```python
from build123d import *

# Parameters (mm, degrees)
SKETCH1_R           = 95.25
BOSS_EXTRUDE1_DEPTH = 19.05
SKETCH2_R           = 56.515
CUT_EXTRUDE1_DEPTH  = 19.05
SKETCH3_R           = 46.355
CUT_EXTRUDE2_DEPTH  = 19.05
SKETCH5_R           = 3.175
CUT_EXTRUDE3_DEPTH  = 38.1
CIRPATTERN1_COUNT   = 3
SKETCH6_R           = 3.175
CUT_EXTRUDE4_DEPTH  = 19.05
CIRPATTERN2_COUNT   = 3


with BuildPart() as part:
    # Sketch1 → Boss-Extrude1 (new body, symmetric)
    with BuildSketch(Plane(origin=(0, 0, 0), x_dir=(1, 0, 0), z_dir=(0, 1, 0))):
        Circle(SKETCH1_R)
    extrude(amount=BOSS_EXTRUDE1_DEPTH, both=True)

    # Sketch2 → Cut-Extrude1 (cut)
    with BuildSketch(Plane(origin=(0, 19.05, 0), x_dir=(-1, 0, 0), z_dir=(0, 1, 0))):
        Circle(SKETCH2_R)
    extrude(amount=-CUT_EXTRUDE1_DEPTH, mode=Mode.SUBTRACT)

    # Sketch3 → Cut-Extrude2 (cut)
    with BuildSketch(Plane.XZ.offset(19.05)):
        Circle(SKETCH3_R)
    extrude(amount=-CUT_EXTRUDE2_DEPTH, mode=Mode.SUBTRACT)

    # Sketch5 → Cut-Extrude3 (cut)
    with BuildSketch(Plane(origin=(0, 19.05, 0), x_dir=(-1, 0, 0), z_dir=(0, 1, 0))):
        with Locations((-76.2, 0)):
            Circle(SKETCH5_R)
    cut_extrude3 = extrude(amount=-CUT_EXTRUDE3_DEPTH, mode=Mode.SUBTRACT)

    # CirPattern1: Cut-Extrude3 ×3 about axis
    cirpattern1_axis = Axis((0, 0, 0), (0, 1, 0))
    for i in range(1, CIRPATTERN1_COUNT):
        add(cut_extrude3.rotate(cirpattern1_axis, i * 360 / CIRPATTERN1_COUNT), mode=Mode.SUBTRACT)

    # Sketch6 → Cut-Extrude4 (cut)
    with BuildSketch(Plane.XZ.offset(19.05)):
        with Locations((44.7675, 77.539584528)):
            Circle(SKETCH6_R)
    cut_extrude4 = extrude(amount=-CUT_EXTRUDE4_DEPTH, mode=Mode.SUBTRACT)

    # CirPattern2: Cut-Extrude4 ×3 about axis
    cirpattern2_axis = Axis((0, 0, 0), (0, 1, 0))
    for i in range(1, CIRPATTERN2_COUNT):
        add(cut_extrude4.rotate(cirpattern2_axis, i * 360 / CIRPATTERN2_COUNT), mode=Mode.SUBTRACT)


solid = part.part
```
Work out the finished part from the listing and answer in its coordinate system (mm). A direction names the side the tool comes from. Coordinates: 2 decimals unless noted, no trailing zeros. Write each loop counter-clockwise with the first axis right and the second up, starting at its lowest first coordinate (ties: lowest second). Pieces come first, ordered by that corner, then holes. Notation, with made-up numbers: (72, 6.5) - (83, 6.5) arc R16 ccw to (83, 24.5) - close; hole circle Ø1 at (-25.5, 35). An arc over 180 degrees is marked (long way). Answer as a JSON object with one key per item and string values.
Q1. Find section A-A (x = 0). Write down the section's boundary in (y, z) (3 decimals).
Results list:
{"outline": "(-19.05, -95.25) - (19.05, -95.25) - (19.05, -56.515) - (0, -56.515) - (0, -46.355) - (-19.05, -46.355) - close; (-19.05, 46.355) - (0, 46.355) - (0, 56.515) - (19.05, 56.515) - (19.05, 95.25) - (-19.05, 95.25) - close"}
Q2. Find section D-D (x = 76.2). Write down the section's boundary in (y, z) (3 decimals).
Results list:
{"outline": "(-19.05, -57.15) - (19.05, -57.15) - (19.05, -3.175) - (-19.05, -3.175) - close; (-19.05, 3.175) - (19.05, 3.175) - (19.05, 57.15) - (-19.05, 57.15) - close"}
Q3. Given pin 1 Ø7.5 at (x, z) = (-38.1, 65.99) entering from -Y; pin 2 Ø3 at (y, z) = (10, -36) entering from +X; pin 3 Ø6 at (y, z) = (15, -60) entering from -X; pin 4 Ø5 at (x, z) = (-89.5, 0.5) entering from -Y, each flat-ended and moving along its own axis, determine where each tip first touches the part or whether it passes through.
Results list:
{"pin 1": "stops at y = -19.05", "pin 2": "stops at x = 88.78", "pin 3": "stops at x = -76.31", "pin 4": "stops at y = 0"}
Q4. Consider L1, parallel to Z at x = -38, y = -1; L2, parallel to Z at x = -38.1, y = -9.5; L3, parallel to Z at x = 0, y = -14 (3 decimals). Determine where each line is inside the solid, lowest interval first. Write a range as from..to.
Results list:
{"L1": "z = -87.34..-69.16, -62.82..-26.55, 26.55..62.82, 69.16..87.34", "L2": "z = -87.3..-69.17, -62.82..-26.4, 26.4..62.82, 69.17..87.3", "L3": "z = -95.25..-46.355, 46.355..95.25"}
Q5. Find section C-C (y = -15). State how many separate pieces and enclosed holes the cut face has, plus the area to 3 significant figures.
Results list:
{"separate pieces": "1", "enclosed holes": "7", "area": "21,600 mm^2"}
Q6. Which of the six approach directions +Z, -Z, +X, -X, +Y, -Y give full straight-line access (tool end or side, diameter ignored) to faces 1 (the flat face through (41, -19.05, -23)), 2 (the flat face through (4.5, 0, 46.3)), 3 (the flat face through (45, 0, 78))?
Results list:
{"face 1": "+Z, -Z, +X, -X, -Y", "face 2": "+Y", "face 3": "-Y"}
Q7. For a pull along Z with two mould halves and no side action, classify faces 4 (the flat face through (-90, 0, 0)), 5 (the flat face through (41, 19.05, 41)), 6 (the cylindrical face through (-75.587, 0.267, 57.958)) as pulls with the +Z half, pulls with the -Z half, needs draft (parallel to the pull), parting line crosses it, or undercut.
Results list:
{"face 4": "undercut", "face 5": "needs draft", "face 6": "parting line crosses it"}
Q8. Find section B-B (z = 0). Write down the section's boundary in (x, y) (3 decimals).
Results list:
{"outline": "(-95.25, -19.05) - (-92.71, -19.05) - (-92.71, 0) - (-86.36, 0) - (-86.36, -19.05) - (-46.355, -19.05) - (-46.355, 0) - (-56.515, 0) - (-56.515, 19.05) - (-95.25, 19.05) - close; (46.355, -19.05) - (73.025, -19.05) - (73.025, 19.05) - (56.515, 19.05) - (56.515, 0) - (46.355, 0) - close; (79.375, -19.05) - (95.25, -19.05) - (95.25, 19.05) - (79.375, 19.05) - close"}
